Autodesk Inventor part; units mm, degrees
ref_plane "YZ Plane" through (0, 0, 0) normal (1, 0, 0) x (0, 1, 0)
ref_plane "XZ Plane" through (0, 0, 0) normal (0, 1, 0) x (-1, 0, 0)
ref_plane "XY Plane" through (0, 0, 0) normal (0, 0, 1) x (1, 0, 0)
sketch "スケッチ1" plane through (0, 0, 0) normal (0, 1, 0) x (-1, 0, 0)
  circle A0 centre (0, 0) radius 86.2565
  line L0 (0, 0) -> (86.2565, 0)
  line L1 (66.4468, 55) -> (-66.4468, 55)
  line L2 (0, 55) -> (14.9, 55)
  line L3 (14.9, 55) -> (14.9, 115)
  line L4 (14.9, 115) -> (0, 115)
  line L5 (0, 115) -> (0, 55)
  line L6 (-14.9, 55) -> (-14.9, 115)
  line L7 (-14.9, 115) -> (0, 115)
  point P0 (14.9, 84.9598)
  point P1 (-14.9, 84.9598)
  dimension "d0" = 172.513
  dimension "d1" = 55
  dimension "d2" = 14.9
  dimension "d3" = 60
extrude "押し出し1" add sketch "スケッチ1" along normal blind 20 contours L1 L3 A0 | A0 L6 L1 | L3 L1 L5 A0 | A0 L5 L4 L3 | L6 L7 L5 A0 | A0 L5 L1 L6
sketch "スケッチ2" plane through (0, 0, 0) normal (0, -1, 0) x (1, 0, 0)
  arc A0 (66.4468, 55) -> (14.9, 84.9598) centre (0, 0) ccw
  circle A1 centre (0, 0) radius 86.2565
  line L0 (-14.9, 115) -> (14.9, 115)
  line L1 (0, 115) -> (7.475, 115)
  line L2 (7.475, 115) -> (7.475, 91.2565)
  line L3 (7.475, 91.2565) -> (0, 91.2565)
  line L4 (0, 91.2565) -> (0, 115)
  line L5 (-7.475, 115) -> (-7.475, 91.2565)
  line L6 (-7.475, 91.2565) -> (0, 91.2565)
  line L7 (14.9, 115) -> (-14.9, 115)
  dimension "d6" = 5
  dimension "d7" = 7.475
extrude "押し出し2" add sketch "スケッチ2" along normal blind 62.1 contours L0 L4 L6 L5 | L0 L2 L3 L4
fillet "フィレット1" radius 5 4 edges at (-14.9, 10, 84.9598) (14.9, 10, 84.9598) (-14.9, 10, 115) (14.9, 10, 115)
fillet "フィレット2" radius 2 4 edges at (-7.475, -31.05, 91.2565) (7.475, -31.05, 91.2565) (-7.475, -31.05, 115) (7.475, -31.05, 115)
properties part number "zigu1"
CAD build for the part. Positions are in the model's coordinates, mm. A direction names the side the tool comes from. Coordinates: 2 decimals unless noted, no trailing zeros. Order: outer loops, then holes, each group sorted by start corner. A loop starts at its lowest first (then second) coordinate and runs counter-clockwise, first axis right, second up. Notation, with made-up numbers: (88.5, -19.5) -> (137.5, -19.5) arc R24 ccw to (137.5, -3.5) -> close; hole circle Ø10 at (61, -33.5). An arc over 180 degrees is marked (long way). Use one line per item in the form item = value. Start each with the question number.
1) Band-saw the part on C-C on x = 38. Give the cut face in (y, z), then the cut area to 3 significant figures.
2) Drop flat-ended pins along their axis: pin 1 (10 mm diameter, centred on y = -35, z = 102, fed in from -X) (3 decimals); pin 2 (6 mm diameter, centred on y = -32.5, z = 98.5, fed in from +X) (3 decimals); pin 3 (5.5 mm diameter, centred on x = -0.5, y = -30.5, fed in from -Z). Give the stop position or say it passes through.
3) Band-saw the part on B-B on z = 63. Give the cut face in (x, y).
4) Drill centre lines: L1, parallel to Y at x = 29.5, z = 61; L2, parallel to X at y = -47.5, z = 93.5 (3 decimals); L3, parallel to X at y = 9, z = 96.5. Where is each one in solid material? Low to high. Write a range as [from, to].
5) Band-saw the part on A-A on y = -16.5. Give the cut face in (x, z) (1 decimal).
6) Band-saw the part on D-D on y = 8. Give the cut face in (x, z).
7) Tool access for faces 1 (the flat face through (-7.475, -31, 103)), 2 (the flat face through (0, -31, 91.256)), 3 (the flat face through (14.9, 10, 99)), 4 (the flat face through (-14.9, 10, 99)): list every direction of +Z, -Z, +X, -X, +Y, -Y with a clear straight run to the whole face (end or side of a thin tool).
Entries:
q1.outline = (0, 55) -> (20, 55) -> (20, 77.44) -> (0, 77.44) -> close
q1.area = 449 mm2
q2.pin_1 = -7.475
q2.pin_2 = 7.475
q2.pin_3 = 91.26
q3.outline = (-58.92, 0) -> (58.92, 0) -> (58.92, 20) -> (-58.92, 20) -> close
q4.L1 = [0, 20]
q4.L2 = [-7.475, 7.475]
q4.L3 = [-14.9, 14.9]
q5.outline = (-7.5, 93.3) arc R2 ccw to (-5.5, 91.3) -> (5.5, 91.3) arc R2 ccw to (7.5, 93.3) -> (7.5, 113) arc R2 ccw to (5.5, 115) -> (-5.5, 115) arc R2 ccw to (-7.5, 113) -> close
q6.outline = (-66.45, 55) -> (66.45, 55) arc R86.26 ccw to (18.81, 84.18) arc R5 cw to (14.9, 89.06) -> (14.9, 110) arc R5 ccw to (9.9, 115) -> (-9.9, 115) arc R5 ccw to (-14.9, 110) -> (-14.9, 89.06) arc R5 cw to (-18.81, 84.18) arc R86.26 ccw to start
q7.face_1 = +Z, -Z, -X, -Y
q7.face_2 = -Z, +X, -X, -Y
q7.face_3 = +Z, +X, +Y, -Y
q7.face_4 = +Z, -X, +Y, -Y
